```python
from build123d import *

# Parameters (mm, degrees)
SKETCH1_W           = 127.75
SKETCH1_H           = 85.6
BOSS_EXTRUDE1_DEPTH = 14.35
FILLET1_R           = 3
CUT_FLANGE_DEPTH    = 8.25
SKETCH5_W           = 80.1
SKETCH5_H           = 0.75
CUT_PAPERSLOT_DEPTH = 123.75
CUT_OPENTOP_REACH   = 80.216
SHELL1_DEPTH        = 11.1
SHELL1_2_DEPTH      = 5.1


# Read off the part's stored shape, not the designer's step: Shell1
with BuildPart() as part:
    # Sketch1 → Boss-Extrude1 (new body)
    with BuildSketch(Plane(origin=(0, 0, 0), x_dir=(1, 0, 0), z_dir=(0, 1, 0))):
        Rectangle(SKETCH1_W, SKETCH1_H)
    extrude(amount=BOSS_EXTRUDE1_DEPTH)

    # Fillet1
    fillet1_edges = [part.edges().sort_by_distance(p)[0] for p in [
        (-63.875, 7.175, -42.8),
        (63.875, 7.175, -42.8),
        (63.875, 7.175, 42.8),
        (-63.875, 7.175, 42.8),
    ]]
    fillet(fillet1_edges, radius=FILLET1_R)

    # Sketch3 → Cut-Flange (cut)
    with BuildSketch(Plane(origin=(0, 14.35, 0), x_dir=(1, 0, 0), z_dir=(0, 1, 0))):
        with BuildLine():
            Line((-63.875, 39.8), (-63.875, -39.8))
            ThreePointArc((-63.875, -39.8), (-62.996320344, -41.921320344), (-60.875, -42.8))
            Line((-60.875, -42.8), (60.875, -42.8))
            ThreePointArc((60.875, -42.8), (62.996320344, -41.921320344), (63.875, -39.8))
            Line((63.875, -39.8), (63.875, 39.8))
            ThreePointArc((63.875, 39.8), (62.996320344, 41.921320344), (60.875, 42.8))
            Line((60.875, 42.8), (-60.875, 42.8))
            ThreePointArc((-60.875, 42.8), (-62.996320344, 41.921320344), (-63.875, 39.8))
        make_face()
        with BuildLine():
            Line((-62.625, 36.600252532), (-62.625, -39.8))
            ThreePointArc((-62.625, -39.8), (-62.112436867, -41.037436867), (-60.875, -41.55))
            Line((-60.875, -41.55), (60.875, -41.55))
            ThreePointArc((60.875, -41.55), (62.112436867, -41.037436867), (62.625, -39.8))
            Line((62.625, -39.8), (62.625, 39.8))
            ThreePointArc((62.625, 39.8), (62.112436867, 41.037436867), (60.875, 41.55))
            Line((60.875, 41.55), (-57.675252532, 41.55))
            Line((-57.675252532, 41.55), (-62.625, 36.600252532))
        make_face(mode=Mode.SUBTRACT)
    extrude(amount=-CUT_FLANGE_DEPTH, mode=Mode.SUBTRACT)

    # Sketch5 → Cut-PaperSlot (cut)
    with BuildSketch(Plane.ZY.offset(62.625)):
        with Locations((0, 12.475)):
            Rectangle(SKETCH5_W, SKETCH5_H)
    extrude(amount=-CUT_PAPERSLOT_DEPTH, mode=Mode.SUBTRACT)

    # Sketch6 → Cut-OpenTop (cut, up to next)
    with BuildSketch(Plane(origin=(0, 14.35, 0), x_dir=(1, 0, 0), z_dir=(0, 1, 0)), mode=Mode.PRIVATE) as cut_opentop_sk1:
        Polygon((-57.675252532, 37.55), (-61.675252532, 37.55), (-62.625, 36.600252532), (-62.625, -37.55), (-60.875, -37.55), (58.625, -37.55), (58.625, 37.55), align=None)
    cut_opentop_tool1 = extrude(cut_opentop_sk1.sketch, amount=-CUT_OPENTOP_REACH, mode=Mode.PRIVATE) & part.part
    add(cut_opentop_tool1.solids().sort_by_distance((-1.997013, 14.35, 0.001844))[0], mode=Mode.SUBTRACT)

    # Shell1 outline → Shell1 (cut)
    with BuildSketch(Plane(origin=(0, 0, 0), x_dir=(1, 0, 0), z_dir=(0, 1, 0))):
        with BuildLine():
            Line((-61.625, 36.186038969), (-61.625, -39.8))
            ThreePointArc((-61.625, -39.8), (-61.405330086, -40.330330086), (-60.875, -40.55))
            Line((-60.875, -40.55), (60.875, -40.55))
            ThreePointArc((60.875, -40.55), (61.405330086, -40.330330086), (61.625, -39.8))
            Line((61.625, -39.8), (61.625, 39.8))
            ThreePointArc((61.625, 39.8), (61.405330086, 40.330330086), (60.875, 40.55))
            Line((60.875, 40.55), (-57.261038969, 40.55))
            Line((-57.261038969, 40.55), (-61.625, 36.186038969))
        make_face()
    extrude(amount=SHELL1_DEPTH, mode=Mode.SUBTRACT)

    # Shell1 2 outline → Shell1 2 (cut)
    with BuildSketch(Plane(origin=(0, 0, 0), x_dir=(1, 0, 0), z_dir=(0, 1, 0))):
        with BuildLine():
            Line((-62.875, 39.8), (-62.875, -39.8))
            ThreePointArc((-62.875, -39.8), (-62.289213562, -41.214213562), (-60.875, -41.8))
            Line((-60.875, -41.8), (60.875, -41.8))
            ThreePointArc((60.875, -41.8), (62.289213562, -41.214213562), (62.875, -39.8))
            Line((62.875, -39.8), (62.875, 39.8))
            ThreePointArc((62.875, 39.8), (62.289213562, 41.214213562), (60.875, 41.8))
            Line((60.875, 41.8), (-60.875, 41.8))
            ThreePointArc((-60.875, 41.8), (-62.289213562, 41.214213562), (-62.875, 39.8))
        make_face()
        with BuildLine():
            ThreePointArc((-60.875, -40.55), (-61.405330086, -40.330330086), (-61.625, -39.8))
            Line((-61.625, -39.8), (-61.625, 36.186038969))
            Line((-61.625, 36.186038969), (-57.261038969, 40.55))
            Line((-57.261038969, 40.55), (60.875, 40.55))
            ThreePointArc((60.875, 40.55), (61.405330086, 40.330330086), (61.625, 39.8))
            Line((61.625, 39.8), (61.625, -39.8))
            ThreePointArc((61.625, -39.8), (61.405330086, -40.330330086), (60.875, -40.55))
            Line((60.875, -40.55), (-60.875, -40.55))
        make_face(mode=Mode.SUBTRACT)
    extrude(amount=SHELL1_2_DEPTH, mode=Mode.SUBTRACT)


solid = part.part
```
Check sheet for the modelled part. Datum: model origin and axes. Units: mm. A direction names the side the tool comes from. Give positions to 0.01 mm unless a question says otherwise; leave off trailing zeros. Order: outer loops, then holes, each group sorted by start corner. A loop starts at its lowest first (then second) coordinate and runs counter-clockwise, first axis right, second up. Notation, with made-up numbers: M 43,7.25 L 101,7.25 A29 cw 101,40.25 Z; hole C 72,-24.5 d3. An arc over 180 degrees is marked long. Answer in a Markdown table with one row per item.
1) Thickness scan on L1, parallel to Z at x = -0.5, y = 7; L2, parallel to X at y = 1.5, z = -8 (3 decimals); L3, parallel to Z at x = -54, y = 12.5. Record the ranges inside material, lowest first. Write a range as [from, to].
Filled sheet:
| item | result |
|---|---|
| L1 | z = [-41.55, -40.55], [40.55, 41.55] |
| L2 | x = [-63.875, -62.875], [62.875, 63.875] |
| L3 | z = [-41.55, -40.05], [40.05, 41.55] |
2) Release check for a two-part mould opening along X. For faces 1 (the flat face through (61.625, 8, 1)), 2 (the flat face through (18, 14.35, 40)), 3 (the cylindrical face through (63.02, 3.09, -41.9)) record: +X half, -X half, draft (parallel to the pull), parting line (faces both ways), or undercut.
Filled sheet:
| item | result |
|---|---|
| face 1 | undercut |
| face 2 | draft |
| face 3 | +X half |
3) Cross-section at A-A, the plane y = 2.5. Enter the section's corners in (x, z) (3 decimals).
Filled sheet:
| item | result |
|---|---|
| outline | M -63.875,-39.8 A3 ccw -60.875,-42.8 L 60.875,-42.8 A3 ccw 63.875,-39.8 L 63.875,39.8 A3 ccw 60.875,42.8 L -60.875,42.8 A3 ccw -63.875,39.8 Z; hole M -62.875,-39.8 A2 ccw -60.875,-41.8 L 60.875,-41.8 A2 ccw 62.875,-39.8 L 62.875,39.8 A2 ccw 60.875,41.8 L -60.875,41.8 A2 ccw -62.875,39.8 Z |
4) Cross-section at D-D, the plane y = 8. Enter the section's corners in (x, z) (3 decimals), plus the area to 3 significant figures.
Filled sheet:
| item | result |
|---|---|
| outline | M -62.625,-36.6 L -57.675,-41.55 L 60.875,-41.55 A1.75 ccw 62.625,-39.8 L 62.625,39.8 A1.75 ccw 60.875,41.55 L -60.875,41.55 A1.75 ccw -62.625,39.8 Z; hole M -61.625,-36.186 L -57.261,-40.55 L 60.875,-40.55 A0.75 ccw 61.625,-39.8 L 61.625,39.8 A0.75 ccw 60.875,40.55 L -60.875,40.55 A0.75 ccw -61.625,39.8 Z |
| area | 408 mm2 |
5) Gauge pin test, flat ends, axial feed: P1, Ø5, axis at x = -50.5, z = 34, coming from the -Y side; P2, Ø6, axis at y = 8, z = 24, coming from the +X side (3 decimals); P3, Ø1.8, axis at x = 14, y = 8, coming from the -Z side; P4, Ø1.8, axis at y = 7.5, z = 6, coming from the -X side (3 decimals). Record the tip position at first contact, or that the pin passes through.
Filled sheet:
| item | result |
|---|---|
| P1 | stops at y = 11.1 |
| P2 | stops at x = 63.875 |
| P3 | stops at z = -41.55 |
| P4 | stops at x = -62.625 |
6) Cross-section at B-B, the plane x = 36. Enter the section's corners in (y, z), plus the area to 3 significant figures.
Filled sheet:
| item | result |
|---|---|
| outline | M 0,-42.8 L 6.1,-42.8 L 6.1,-41.55 L 14.35,-41.55 L 14.35,-37.55 L 12.85,-37.55 L 12.85,-40.05 L 12.1,-40.05 L 12.1,40.05 L 12.85,40.05 L 12.85,37.55 L 14.35,37.55 L 14.35,41.55 L 6.1,41.55 L 6.1,42.8 L 0,42.8 L 0,41.8 L 5.1,41.8 L 5.1,40.55 L 11.1,40.55 L 11.1,-40.55 L 5.1,-40.55 L 5.1,-41.8 L 0,-41.8 Z |
| area | 122 mm2 |
7) Cross-section at C-C, the plane z = 18.5. Enter the section's corners in (x, y) (3 decimals).
Filled sheet:
| item | result |
|---|---|
| outline | M -63.875,0 L -62.875,0 L -62.875,5.1 L -61.625,5.1 L -61.625,11.1 L 61.625,11.1 L 61.625,5.1 L 62.875,5.1 L 62.875,0 L 63.875,0 L 63.875,6.1 L 62.625,6.1 L 62.625,14.35 L 58.625,14.35 L 58.625,12.85 L 61.125,12.85 L 61.125,12.1 L -62.625,12.1 L -62.625,6.1 L -63.875,6.1 Z |
8) Access from +Z, -Z, +X, -X, +Y, -Y to the whole of each face (thin tool, end or side, straight path). Record for faces 4 (the flat face through (-1, 10, 41.55)), 5 (the flat face through (-1, 12.85, 38)), 6 (the flat face through (-62.875, 3, -1)), 7 (the flat face through (-60.115, 10.283, -39.11)).
Filled sheet:
| item | result |
|---|---|
| face 4 | +Z, +X, -X, +Y |
| face 5 | -X |
| face 6 | -Y |
| face 7 | -Z, -X, +Y |
